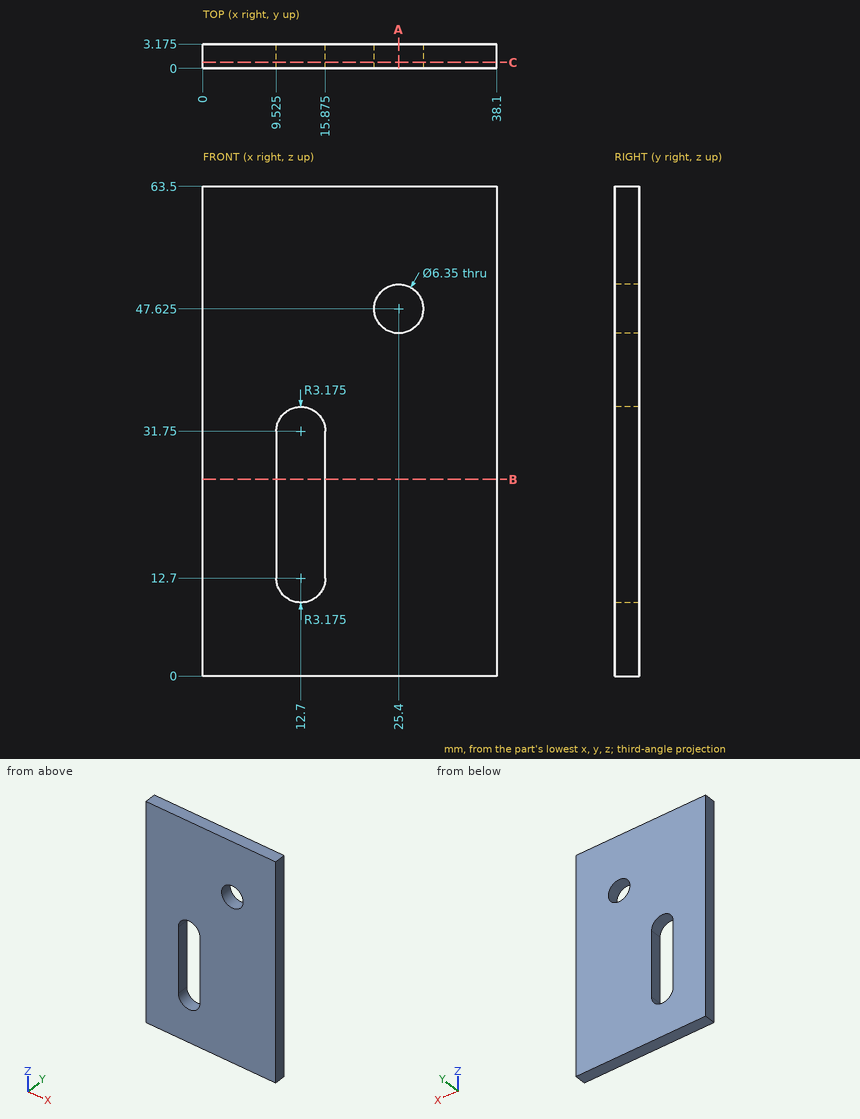
Verification items for this drawing (mm, ordinates from the low corner). Round coordinates to 2 decimals unless told otherwise and drop trailing zeros. Order: outer loops, then holes, each group sorted by start corner. A loop starts at its lowest first (then second) coordinate and runs counter-clockwise, first axis right, second up. Notation, with made-up numbers: M -10,48.5 L -1,48.5 A15 cw -1,52.5 Z; hole C 41,9.25 d1. An arc over 180 degrees is marked long. Answer in a Markdown table with one row per item. Add a question column.
Item 1: Sectioned sample at A-A, the plane x = 25.4. Enter the section's corners in (y, z) (3 decimals).
Item 2: Sectioned sample at B-B, the plane z = 25.5. Enter the section's corners in (x, y) (3 decimals).
Item 3: Sectioned sample at C-C, the plane y = 0.8. Enter the section's corners in (x, z) (3 decimals), plus the area to 3 significant figures.
Item 4: Depth check by flat-ended pin: pin 1 Ø4 at (x, z) = (13.5, 30.5) entering from -Y. Enter the tip coordinate at first touch or a pass-through.
Item 5: Material ranges on L1, parallel to Z at x = 25.4, y = 1.85; L2, parallel to X at y = 1.8, z = 27.5 (3 decimals); L3, parallel to X at y = 1.75, z = 47, recorded low to high. Write a range as [from, to].
Filled in:
| question | item | result |
|---|---|---|
| 1 | outline | M 0,0 L 3.175,0 L 3.175,44.45 L 0,44.45 Z; M 0,50.8 L 3.175,50.8 L 3.175,63.5 L 0,63.5 Z |
| 2 | outline | M 0,0 L 9.525,0 L 9.525,3.175 L 0,3.175 Z; M 15.875,0 L 38.1,0 L 38.1,3.175 L 15.875,3.175 Z |
| 3 | outline | M 0,0 L 38.1,0 L 38.1,63.5 L 0,63.5 Z; hole M 9.525,12.7 A3.175 ccw 15.875,12.7 L 15.875,31.75 A3.175 ccw 9.525,31.75 Z; hole C 25.4,47.625 d6.35 |
| 3 | area | 2,240 mm² |
| 4 | pin 1 | passes through |
| 5 | L1 | z = [0, 44.45], [50.8, 63.5] |
| 5 | L2 | x = [0, 9.525], [15.875, 38.1] |
| 5 | L3 | x = [0, 22.29], [28.51, 38.1] |
